The listing builds one solid part. Answer for the finished solid, in the listing's coordinates (mm). A direction names the side the tool comes from. Coordinates: 2 decimals unless noted, no trailing zeros. Order: outer loops, then holes, each group sorted by start corner. A loop starts at its lowest first (then second) coordinate and runs counter-clockwise, first axis right, second up.
```python
from build123d import *

# Parameters (mm, degrees)
F0_W     = 12.25
F0_H     = 15
F1_DEPTH = 15
F2_R     = 7.49999
F3_R     = 1
F4_DEPTH = 25
F6_DEPTH = 4.5
F8_DEPTH = 3


# Not quite as in the source:
# - a fillet or chamfer is up to 0.001 mm smaller than in the source, because OpenCascade refuses the exact size


with BuildPart() as f1:
    # F0 (on Front) → F1 (new body)
    with BuildSketch(Plane.XZ):
        with Locations((-33.7760131806, 25.872811313)):
            Rectangle(F0_W, F0_H)
    extrude(amount=F1_DEPTH)

    # F2 (radius 7.5 in the source; OpenCascade refuses exactly that, so slightly less here)
    f2_edges = [f1.edges().sort_by_distance(p)[0] for p in [
        (-33.776013, 0, 18.372811),
        (-33.776013, 0, 33.372811),
    ]]
    fillet(f2_edges, radius=F2_R)

    # F3 (on face) → F4 (cut)
    with BuildSketch(Plane(origin=(-39.9010131806, 0, 0), x_dir=(0, -1, 0), z_dir=(-1, 0, 0))):
        with Locations((7.5, 25.872811313)):
            Circle(F3_R)
    extrude(amount=-F4_DEPTH, mode=Mode.SUBTRACT)

    # F5 (on face) → F6 (cut)
    with BuildSketch(Plane.YZ.offset(-27.6510131806)):
        Polygon((-9, 30.372811313), (-15, 30.372811313), (-15, 21.372811313), (-9, 21.372811313), (-9, 25.872811313), align=None)
    extrude(amount=-F6_DEPTH, mode=Mode.SUBTRACT)

    # F7 (on face) → F8 (join)
    with BuildSketch(Plane.XZ.offset(15)):
        with BuildLine():
            Line((-27.6510131806, 30.372811313), (-32.1510131806, 30.372811313))
            Line((-32.1510131806, 30.372811313), (-32.1510131806, 21.372811313))
            Line((-32.1510131806, 21.372811313), (-27.6510131806, 21.372811313))
            Line((-27.6510131806, 21.372811313), (-27.6510131806, 21.872811313))
            ThreePointArc((-27.6510131806, 21.872811313), (-31.6510131806, 25.872811313), (-27.6510131806, 29.872811313))
            Line((-27.6510131806, 29.872811313), (-27.6510131806, 30.372811313))
        make_face()
    extrude(amount=-F8_DEPTH)


solid = f1.part
```
(1) Consider line 1 (Z direction, x = -34.5, y = -7.5); line 2 (Z direction, x = -31.5, y = -9.5); line 3 (X direction, y = -10.5, z = 27.75). Determine where each line is inside the solid, lowest interval first.
(2) Find section D-D (y = -7.25). Write down the section's boundary in (x, z).
(3) For faces 1 (the face through (-30, -10, 30.373)), 2 (the face through (-33.69, -2.255, 20.512)), 3 (the face through (-31.65, -13.52, 25.78)), determine the directions among +Z, -Z, +X, -X, +Y, -Y from which every point of the face is accessible in a straight line to the end or side of a thin tool.
(4) Each of these flat-tipped pins is pushed along its axis until it touches: pin 1 Ø1.4 at (x, z) = (-30.5, 26) entering from -Y; pin 2 Ø3.5 at (y, z) = (-11, 24.5) entering from +X; pin 3 Ø2.5 at (y, z) = (-7.5, 25.87) entering from -X; pin 4 Ø3 at (y, z) = (-13, 25) entering from +X. Where does it stop, or does it pass through?
(5) Find section C-C (z = 25.5). Write down the section's boundary in (x, y).
(6) The mould has two halves that part along Y. Classify faces 4 (the face through (-30, -9, 26)), 5 (the face through (-35, -15, 26)), 6 (the face through (-33.69, -2.255, 31.234)), 7 (the face through (-34, -11, 33.373)): released by +Y, released by -Y, zero draft, split by the parting line, or undercut.
(7) Find section B-B (y = -9.5). Write down the section's boundary in (x, z), and give its area (3 significant figures).
Findings below:
1. line 1: z = 18.37 to 24.87, 26.87 to 33.37
1. line 2: z = 18.37 to 21.37, 30.37 to 33.37
1. line 3: x = -39.9 to -32.15
2. outline: (-39.9, 18.38) - (-27.65, 18.38) - (-27.65, 24.9) - (-39.9, 24.9) - close; (-39.9, 26.84) - (-27.65, 26.84) - (-27.65, 33.37) - (-39.9, 33.37) - close
3. face 1: +X
3. face 2: -Z, +X, -X, +Y
3. face 3: +X, -Y
4. pin 1: stops at y = -9
4. pin 2: stops at x = -30.5
4. pin 3: stops at x = -39.9
4. pin 4: stops at x = -30.87
5. outline: (-39.9, -15) - (-31.63, -15) - (-31.63, -12) - (-32.15, -12) - (-32.15, -9) - (-27.65, -9) - (-27.65, -8.43) - (-39.9, -8.43) - close; (-39.9, -6.57) - (-27.65, -6.57) - (-27.65, -0.01) - (-39.9, -0.01) - close
6. face 4: undercut
6. face 5: released by -Y
6. face 6: released by +Y
6. face 7: zero draft
7. outline: (-39.9, 18.37) - (-27.65, 18.37) - (-27.65, 21.37) - (-32.15, 21.37) - (-32.15, 30.37) - (-27.65, 30.37) - (-27.65, 33.37) - (-39.9, 33.37) - close
7. area: 143 mm2
